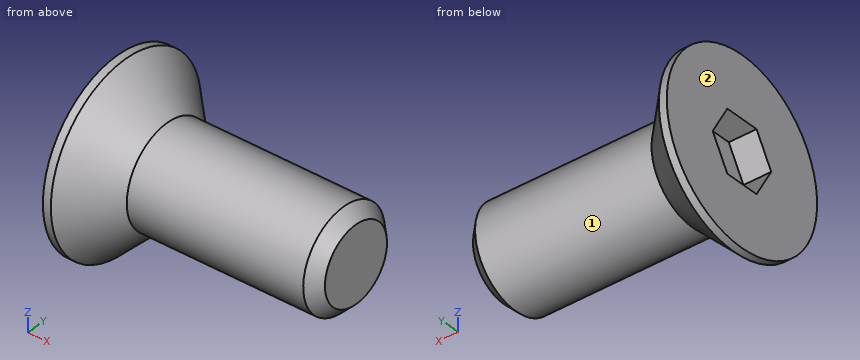
Autodesk Inventor part; units mm, degrees
ref_plane "YZ Plane" through (0, 0, 0) normal (1, 0, 0) x (0, 1, 0)
ref_plane "XZ Plane" through (0, 0, 0) normal (0, 1, 0) x (-1, 0, 0)
ref_plane "XY Plane" through (0, 0, 0) normal (0, 0, 1) x (1, 0, 0)
sketch "スケッチ1" plane through (0, 0, 0) normal (0, 1, 0) x (-1, 0, 0)
  line L0 (0, 0) -> (4.75, 0)
  line L1 (4.75, 0) -> (4.75, 1.25)
  line L2 (0, 0.95) -> (0, 0)
  line L3 (5.8, 2.3) -> (6, 2.3)
  line L4 (6, 2.3) -> (6, 0)
  line L5 (6, 0) -> (4.75, 0)
  line L6 (4.75, 1.25) -> (0.3, 1.25)
  line L7 (0.3, 1.25) -> (0, 0.95)
  line L8 (4.75, 1.25) -> (5.8, 2.3)
  line L9 (5.8, 2.3) -> (6, 2.3)
  point P0 (6, 1.15)
  dimension "d1" = 6
  dimension "d4" = 45
  dimension "d5" = 1.25
  dimension "d6" = 0.3
  dimension "d8" = 45
  dimension "d9" = 0.2
  dimension "d10" = 1.25
revolve "回転1" add sketch "スケッチ1" angle 360 about axis through (0, 0, 0) along (-1, 0, 0)
sketch "スケッチ2" plane through (-6, 0, 0) normal (-1, 0, 0) x (0, 0, 1)
  circle A0 centre (0, 0) radius 0.95
  line L0 (0, 0.8949) -> (0.775, 0.4474)
  line L1 (0.775, 0.4474) -> (0.775, -0.4474)
  line L2 (0.775, -0.4474) -> (0, -0.8949)
  line L3 (0, -0.8949) -> (-0.775, -0.4474)
  line L4 (-0.775, -0.4474) -> (-0.775, 0.4474)
  line L5 (-0.775, 0.4474) -> (0, 0.8949)
  point P0 (0, 0)
  dimension "d12" = 1.55
extrude "押し出し1" cut sketch "スケッチ2" against normal blind 0.7 contours L0 L1 L2 L3 L4 L5
thread "ねじ1"
properties part number "CSHCS-SUS-M2_5-6"
Could you check a few things on this model? Use its own coordinates, in mm. Face numbers are marked on the shaded views. A direction names the side the tool comes from. Round coordinates to 2 decimals unless told otherwise and drop trailing zeros. Loops run counter-clockwise (first coordinate to the right, second up) from the corner with the lowest first, then second, coordinate; pieces in that order, holes last. Notation, with made-up numbers: M -15.5,47 L 12.5,47 A10 ccw 12.5,64 Z; hole C 32,59.25 d4. An arc over 180 degrees is marked long. Write item = value, one per line.
1. I need wall thicknesses on probe 1 along Y at (x, z) = (-4.05, 0.75); probe 2 along Z at (x, y) = (-5.5, 0.5); probe 3 along X at (y, z) = (-0.6, -1.55). Which ranges of each line are inside material? Lowest first, please.
Results below:
probe_1 = -1 to 1
probe_2 = -1.94 to -0.68, 0.68 to 1.94
probe_3 = -6 to -5.16
2. I want a section at B-B, the plane x = -3.25. Write out the boundary of the cut face in (y, z).
Results below:
outline = C 0,0 d2.5
3. Which directions (+Z, -Z, +X, -X, +Y, -Y) give clear straight access to the entire face, cutting with the end or side of a thin tool? Please do the marked faces 1 and 2.
Results below:
face_1 = +X
face_2 = +Z, -Z, -X, +Y, -Y
4. Will this pin go through, and if not, where does the flat tip stop? P1, Ø1.5, axis at x = -2, z = -1, coming from the -Y side.
Results below:
P1 = -1.22
5. I want a section at A-A, the plane y = 0. Write out the boundary of the cut face in (x, z) (3 decimals), and give its area (3 significant figures).
Results below:
outline = M -6,-2.3 L -5.8,-2.3 L -4.75,-1.25 L -0.3,-1.25 L 0,-0.95 L 0,0.95 L -0.3,1.25 L -4.75,1.25 L -5.8,2.3 L -6,2.3 L -6,0.775 L -5.3,0.775 L -5.3,-0.775 L -6,-0.775 Z
area = 15.3 mm²
